For this review, take the finished solid that the model builds, in its own axes (mm). A direction names the side the tool comes from. Round coordinates to 2 decimals unless told otherwise and drop trailing zeros. Order: outer loops, then holes, each group sorted by start corner. A loop starts at its lowest first (then second) coordinate and runs counter-clockwise, first axis right, second up.
```python
from build123d import *

# Parameters (mm, degrees)
SKETCH1_R           = 8.89
BOSS_EXTRUDE1_DEPTH = 5.08
BOSS_EXTRUDE2_DEPTH = 7.62
SKETCH3_R           = 5.55625
BOSS_EXTRUDE3_DEPTH = 19.05
SKETCH4_R           = 12.7
BOSS_EXTRUDE4_DEPTH = 27.94
SKETCH5_R           = 1.397
CUT_EXTRUDE1_DEPTH  = 20.32


with BuildPart() as part:
    # Sketch1 → Boss-Extrude1 (new body)
    with BuildSketch(Plane(origin=(0, 0, 0), x_dir=(1, 0, 0), z_dir=(0, 1, 0))):
        Circle(SKETCH1_R)
    extrude(amount=BOSS_EXTRUDE1_DEPTH)

    # Sketch2 → Boss-Extrude2 (add)
    with BuildSketch(Plane.XZ):
        Polygon((-5.715, 9.525), (5.715, 9.525), (10.795, 0), (5.715, -9.525), (-5.715, -9.525), (-10.795, 0), align=None)
    extrude(amount=BOSS_EXTRUDE2_DEPTH)

    # Sketch3 → Boss-Extrude3 (add)
    with BuildSketch(Plane(origin=(0, -7.62, 0), x_dir=(-1, 0, 0), z_dir=(0, -1, 0))):
        Circle(SKETCH3_R)
    extrude(amount=BOSS_EXTRUDE3_DEPTH)

    # Sketch4 → Boss-Extrude4 (add)
    with BuildSketch(Plane(origin=(0, 5.08, 0), x_dir=(1, 0, 0), z_dir=(0, 1, 0))):
        Circle(SKETCH4_R)
    extrude(amount=BOSS_EXTRUDE4_DEPTH)

    # Sketch5 → Cut-Extrude1 (cut)
    with BuildSketch(Plane(origin=(0, 33.02, 0), x_dir=(1, 0, 0), z_dir=(0, 1, 0))):
        with Locations((4.171282729, 8.897519777)):
            Circle(SKETCH5_R)
        with Locations((9.139929654, 3.609313469)):
            Circle(SKETCH5_R)
        with Locations((9.125005102, -3.646880814)):
            Circle(SKETCH5_R)
        with Locations((4.134646728, -8.914603425)):
            Circle(SKETCH5_R)
        with Locations((-3.110139008, -9.321614299)):
            Circle(SKETCH5_R)
        with Locations((-8.659113, -4.645989651)):
            Circle(SKETCH5_R)
        with Locations((-9.486682104, 2.562873477)):
            Circle(SKETCH5_R)
    extrude(amount=-CUT_EXTRUDE1_DEPTH, mode=Mode.SUBTRACT)


solid = part.part
```
Q1. Mouldability with a two-part tool opening along X and no side actions: class faces 1 (the face through (4, 12.7, 9)), 2 (the face through (8.22, -3.76, 4.83)), 3 (the face through (9, 0, 1)) as +X half, -X half, draft (parallel to the pull), parting line (faces both ways), or undercut.
Q2. Clearance check with flat-ended pins moving along their axes: pin 1 (1 mm diameter, centred on x = 3.5, y = 25.5, fed in from -Z); pin 2 (8.5 mm diameter, centred on x = 0, y = -2, fed in from +Z) (3 decimals); pin 3 (6 mm diameter, centred on x = -8.5, z = -2.5, fed in from -Y); pin 4 (12 mm diameter, centred on x = -4, y = 16, fed in from +Z). State where each tip first meets the part, or that it passes through.
Q3. Tool access review of faces 4 (the face through (-5.3, -17.01, -1.67)), 5 (the face through (0, -4, -9.525)), 6 (the face through (-10, 12.7, -3)): name each direction out of +Z, -Z, +X, -X, +Y, -Y from which nothing blocks a thin tool from reaching the whole face with its end or side.
Q4. Wall thickness on line 1 (X direction, y = 13.5, z = -2.75); line 2 (Y direction, x = -7.5, z = -3); line 3 (Z direction, x = -2.5, y = -7.5) (3 decimals): over which ranges is each line inside the solid? List them lowest first.
Q5. Take a section at C-C, the plane y = 2.5. State the section outline as (x, z) points.
Q6. Take a section at D-D, the plane x = 7. State the section outline as (y, z) points, plus the area to 3 significant figures.
Q7. Take a section at A-A, the plane x = 0. State the section outline as (y, z) points (3 decimals), plus the area to 3 significant figures.
Q8. Take a section at B-B, the plane y = 14.5. State the section outline as (x, z) points (3 decimals), plus the area to 3 significant figures.
Working result:
1. face 1: undercut
1. face 2: +X half
1. face 3: draft
2. pin 1: stops at z = -12.34
2. pin 2: stops at z = 9.525
2. pin 3: stops at y = -7.62
2. pin 4: stops at z = 12.7
3. face 4: -Y
3. face 5: -Z, +X, -X, -Y
3. face 6: +Y
4. line 1: x = -12.4 to -10.87, -8.1 to 8.04, 10.24 to 12.4
4. line 2: y = -7.62 to 33.02
4. line 3: z = -9.525 to 9.525
5. outline: circle Ø17.78 at (0, 0)
6. outline: (-7.62, -7.12) - (0, -7.12) - (0, -5.48) - (5.08, -5.48) - (5.08, -10.6) - (33.02, -10.6) - (33.02, 10.6) - (5.08, 10.6) - (5.08, 5.48) - (0, 5.48) - (0, 7.12) - (-7.62, 7.12) - close
6. area: 756 mm2
7. outline: (-26.67, -5.556) - (-7.62, -5.556) - (-7.62, -9.525) - (0, -9.525) - (0, -8.89) - (5.08, -8.89) - (5.08, -12.7) - (33.02, -12.7) - (33.02, 12.7) - (5.08, 12.7) - (5.08, 8.89) - (0, 8.89) - (0, 9.525) - (-7.62, 9.525) - (-7.62, 5.556) - (-26.67, 5.556) - close
7. area: 1,160 mm2
8. outline: circle Ø25.4 at (0, 0); hole circle Ø2.794 at (-9.487, -2.563); hole circle Ø2.794 at (-8.659, 4.646); hole circle Ø2.794 at (-3.11, 9.322); hole circle Ø2.794 at (4.135, 8.915); hole circle Ø2.794 at (4.171, -8.898); hole circle Ø2.794 at (9.125, 3.647); hole circle Ø2.794 at (9.14, -3.609)
8. area: 464 mm2
